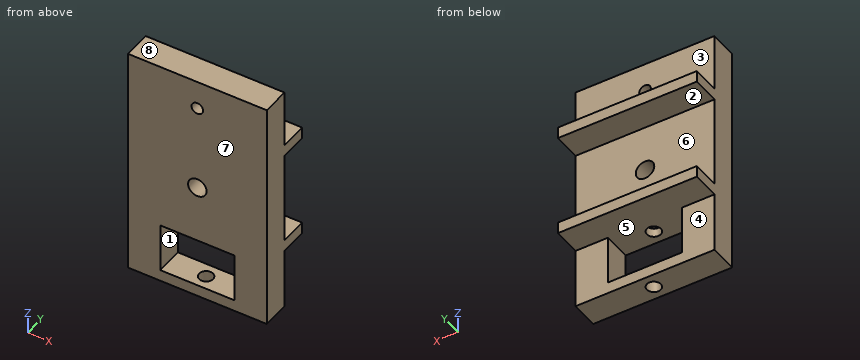
from build123d import *

# Parameters (mm, degrees)
SKETCH1_W           = 30
SKETCH1_H           = 20
SKETCH1_H_2         = 2.5
SKETCH1_W_2         = 16
SKETCH1_W_3         = 7
SKETCH1_H_3         = 10.6
BOSS_EXTRUDE1_DEPTH = 6
SKETCH1_3_W         = 7
SKETCH1_3_H         = 2.5
SKETCH1_3_W_2       = 16
SKETCH1_3_W_3       = 30
BOSS_EXTRUDE2_DEPTH = 12
SKETCH3_R           = 1.5
CUT_EXTRUDE2_DEPTH  = 15
CUT_EXTRUDE1_DEPTH  = 38.976966704
SKETCH5_W           = 30
SKETCH5_H           = 12.5
SKETCH5_R           = 1.25
BOSS_EXTRUDE3_DEPTH = 6


with BuildPart() as part:
    # Sketch1 → Boss-Extrude1 (new body)
    with BuildSketch(Plane(origin=(0, 0, 0), x_dir=(1, 0, 0), z_dir=(0, 1, 0))):
        with Locations((-15, -10)):
            Rectangle(SKETCH1_W, SKETCH1_H)
        with Locations((-15, -21.25)):
            Rectangle(SKETCH1_W, SKETCH1_H_2)
        with Locations((-15, 1.25)):
            Rectangle(SKETCH1_W_2, SKETCH1_H_2)
        with Locations((-3.5, 1.25)):
            Rectangle(SKETCH1_W_3, SKETCH1_H_2)
        with Locations((-3.5, 7.8)):
            Rectangle(SKETCH1_W_3, SKETCH1_H_3)
        with Locations((-3.5, 14.35)):
            Rectangle(SKETCH1_W_3, SKETCH1_H_2)
        with Locations((-15, 14.35)):
            Rectangle(SKETCH1_W_2, SKETCH1_H_2)
        with Locations((-26.5, 14.35)):
            Rectangle(SKETCH1_W_3, SKETCH1_H_2)
        with Locations((-26.5, 7.8)):
            Rectangle(SKETCH1_W_3, SKETCH1_H_3)
        with Locations((-26.5, 1.25)):
            Rectangle(SKETCH1_W_3, SKETCH1_H_2)
    extrude(amount=BOSS_EXTRUDE1_DEPTH)

    # Sketch1_3 → Boss-Extrude2 (add)
    with BuildSketch(Plane(origin=(0, 0, 0), x_dir=(1, 0, 0), z_dir=(0, 1, 0))):
        with Locations((-3.5, 1.25)):
            Rectangle(SKETCH1_3_W, SKETCH1_3_H)
        with Locations((-15, 1.25)):
            Rectangle(SKETCH1_3_W_2, SKETCH1_3_H)
        with Locations((-15, -21.25)):
            Rectangle(SKETCH1_3_W_3, SKETCH1_3_H)
        with Locations((-26.5, 1.25)):
            Rectangle(SKETCH1_3_W, SKETCH1_3_H)
    extrude(amount=BOSS_EXTRUDE2_DEPTH)

    # Sketch3 → Cut-Extrude2 (cut)
    with BuildSketch(Plane(origin=(0, 0, -15.6), x_dir=(-1, 0, 0), z_dir=(0, 0, -1))):
        with Locations((15, 3)):
            Circle(SKETCH3_R)
    extrude(amount=-CUT_EXTRUDE2_DEPTH, mode=Mode.SUBTRACT)

    # Sketch2 → Cut-Extrude1 (cut, through all)
    with BuildSketch(Plane(origin=(0, 6, 0), x_dir=(1, 0, 0), z_dir=(0, 1, 0))):
        with BuildLine():
            ThreePointArc((-13, -10), (-15, -8), (-17, -10))
            Line((-17, -10), (-13, -10))
        make_face()
        with BuildLine():
            Line((-13, -10), (-17, -10))
            ThreePointArc((-17, -10), (-15, -12), (-13, -10))
        make_face()
    extrude(amount=-CUT_EXTRUDE1_DEPTH, mode=Mode.SUBTRACT)

    # Sketch5 → Boss-Extrude3 (add)
    with BuildSketch(Plane.XZ):
        with Locations((-15, 28.75)):
            Rectangle(SKETCH5_W, SKETCH5_H)
        with Locations(Location((-15, 28.75, 0), (0, 0, 270))):
            Circle(SKETCH5_R, mode=Mode.SUBTRACT)
    extrude(amount=-BOSS_EXTRUDE3_DEPTH)


solid = part.part
Build history of the part. All positions in model axes, mm. Face numbers are marked on the shaded views. A direction names the side the tool comes from. Round coordinates to 2 decimals unless told otherwise and drop trailing zeros. Loops run counter-clockwise (first coordinate to the right, second up) from the corner with the lowest first, then second, coordinate; pieces in that order, holes last. Notation, with made-up numbers: (9, 67) -> (48, 67) arc R19 ccw to (48, 75) -> close; hole circle Ø4 at (6, 47). An arc over 180 degrees is marked (long way). One line per item, written item: value. Start each with the question number.
Q1. Probe line 1 along Z through (x, y) = (-9, 9.75); line 2 along Y through (x, z) = (-15, -14.9); line 3 along Z through (x, y) = (-12.75, 4). List the from-to ranges inside material, lowest first.
Q2. 3-axis set-ups, long thin cutter, end or side, ignore diameter. For the marked faces 1, 2, 3 and 4: which of +Z, -Z, +X, -X, +Y, -Y reach the whole face in a straight line?
Q3. Cut at A-A on z = 28.75. List the corners of the cut face in (x, y).
Q4. Cut at B-B on x = -18. List the corners of the cut face in (y, z), plus the area to 3 significant figures.
Q5. Two-plate mould, pull along Z, no slides. Class the marked faces 5, 6, 7 and 8: released by +Z, released by -Z, zero draft, split by the parting line, or undercut.
Q6. Cut at D-D on x = -15. Count the separate pieces of the cut face and the enclosed holes in it, plus the area to 3 significant figures.
Q7. Cut at C-C on y = 3. List the corners of the cut face in (x, z).
Q8. Drop flat-ended pins along their axis: pin 1 Ø3 at (x, y) = (-21.5, 10) entering from +Z; pin 2 Ø1.8 at (x, y) = (-15, 3) entering from -Z; pin 3 Ø6 at (x, z) = (-21.5, 10.5) entering from +Y; pin 4 Ø1.5 at (x, z) = (-15, 28.75) entering from +Y. Give the stop position or say it passes through.
Computed:
1. line 1: -2.5 to 0, 20 to 22.5
1. line 2: 0 to 1.5, 4.5 to 6
1. line 3: -15.6 to -13.1, -2.5 to 35
2. face 1: +Y, -Y
2. face 2: +X, -X, +Y
2. face 3: +Z, +X, -X, +Y
2. face 4: -Z, +X, -X, +Y
3. outline: (-30, 0) -> (-16.25, 0) -> (-16.25, 6) -> (-30, 6) -> close; (-13.75, 0) -> (0, 0) -> (0, 6) -> (-13.75, 6) -> close
4. outline: (0, -15.6) -> (6, -15.6) -> (6, -13.1) -> (0, -13.1) -> close; (0, -2.5) -> (12, -2.5) -> (12, 0) -> (6, 0) -> (6, 20) -> (12, 20) -> (12, 22.5) -> (6, 22.5) -> (6, 35) -> (0, 35) -> close
4. area: 270 mm²
5. face 5: undercut
5. face 6: undercut
5. face 7: zero draft
5. face 8: released by +Z
6. separate pieces: 5
6. enclosed holes: 0
6. area: 218 mm²
7. outline: (-30, -15.6) -> (-16.5, -15.6) -> (-16.5, -13.1) -> (-23, -13.1) -> (-23, -2.5) -> (-16.5, -2.5) -> (-16.5, -0.6) -> (-13.5, -0.6) -> (-13.5, -2.5) -> (-7, -2.5) -> (-7, -13.1) -> (-13.5, -13.1) -> (-13.5, -15.6) -> (0, -15.6) -> (0, 35) -> (-30, 35) -> close; hole circle Ø4 at (-15, 10); hole circle Ø2.5 at (-15, 28.75)
8. pin 1: z = 22.5
8. pin 2: z = -0.6
8. pin 3: y = 6
8. pin 4: through
